For this review, take the finished solid that the model builds, in its own axes (mm). Coordinates: 2 decimals unless noted, no trailing zeros.
```python
from build123d import *

# Parameters (mm, degrees)
MODEL_R             = 2.75
BOSS_EXTRUDE1_DEPTH = 250


with BuildPart() as part:
    # Model → Boss-Extrude1 (new body)
    with BuildSketch(Plane.XY):
        with BuildLine():
            Line((1.499999935, 19.99999323), (6.799999935, 19.99999323))
            Line((6.799999935, 19.99999323), (6.799999935, 18.69999323))
            Line((6.799999935, 18.69999323), (3.999999935, 18.69999323))
            Line((3.999999935, 18.69999323), (3.999999935, 17.19999323))
            Line((3.999999935, 17.19999323), (6.745762647, 14.5))
            Line((6.745762647, 14.5), (9.565216879, 14.5))
            Line((9.565216879, 14.5), (10, 14.25))
            Line((10, 14.25), (10.434782606, 14.5))
            Line((10.434782606, 14.5), (13.254244108, 14.5))
            Line((13.254244108, 14.5), (15.999999935, 17.19999323))
            Line((15.999999935, 17.19999323), (15.999999935, 18.69999323))
            Line((15.999999935, 18.69999323), (13.199999935, 18.69999323))
            Line((13.199999935, 18.69999323), (13.199999935, 19.99999323))
            Line((13.199999935, 19.99999323), (18.499999935, 19.99999323))
            ThreePointArc((18.499999935, 19.99999323), (19.560660107, 19.560653402), (19.999999935, 18.49999323))
            Line((19.999999935, 18.49999323), (19.999999935, 13.19999323))
            Line((19.999999935, 13.19999323), (18.699999935, 13.19999323))
            Line((18.699999935, 13.19999323), (18.699999935, 15.99999323))
            Line((18.699999935, 15.99999323), (17.199999935, 15.99999323))
            Line((17.199999935, 15.99999323), (14.500000065, 13.254230518))
            Line((14.500000065, 13.254230518), (14.500000065, 10.434776138))
            Line((14.500000065, 10.434776138), (14.250000065, 9.99999323))
            Line((14.250000065, 9.99999323), (14.500000065, 9.565210911))
            Line((14.500000065, 9.565210911), (14.500000065, 6.745755942))
            Line((14.500000065, 6.745755942), (17.199999935, 3.99999323))
            Line((17.199999935, 3.99999323), (18.699999935, 3.99999323))
            Line((18.699999935, 3.99999323), (18.699999935, 6.79999323))
            Line((18.699999935, 6.79999323), (19.999999935, 6.79999323))
            Line((19.999999935, 6.79999323), (19.999999935, 1.49999323))
            ThreePointArc((19.999999935, 1.49999323), (19.560660107, 0.439333058), (18.499999935, -6.77e-06))
            Line((18.499999935, -6.77e-06), (13.199999935, -6.77e-06))
            Line((13.199999935, -6.77e-06), (13.199999935, 1.29999323))
            Line((13.199999935, 1.29999323), (15.999999935, 1.29999323))
            Line((15.999999935, 1.29999323), (15.999999935, 2.798703306))
            Line((15.999999935, 2.798703306), (13.254126104, 5.49999323))
            Line((13.254126104, 5.49999323), (10.434782606, 5.49999323))
            Line((10.434782606, 5.49999323), (10, 5.74999323))
            Line((10, 5.74999323), (9.565216879, 5.49999323))
            Line((9.565216879, 5.49999323), (6.745762647, 5.49999323))
            Line((6.745762647, 5.49999323), (3.999999935, 2.79999323))
            Line((3.999999935, 2.79999323), (3.999999935, 1.29999323))
            Line((3.999999935, 1.29999323), (6.799999935, 1.29999323))
            Line((6.799999935, 1.29999323), (6.799999935, -6.77e-06))
            Line((6.799999935, -6.77e-06), (1.499999935, -6.77e-06))
            ThreePointArc((1.499999935, -6.77e-06), (0.439339764, 0.439333058), (-6.5e-08, 1.49999323))
            Line((-6.5e-08, 1.49999323), (-6.5e-08, 6.79999323))
            Line((-6.5e-08, 6.79999323), (1.299999935, 6.79999323))
            Line((1.299999935, 6.79999323), (1.299999935, 3.99999323))
            Line((1.299999935, 3.99999323), (2.799999935, 3.99999323))
            Line((2.799999935, 3.99999323), (5.499999935, 6.745755942))
            Line((5.499999935, 6.745755942), (5.499999935, 9.565210911))
            Line((5.499999935, 9.565210911), (5.749999935, 9.99999323))
            Line((5.749999935, 9.99999323), (5.499999935, 10.434776138))
            Line((5.499999935, 10.434776138), (5.499999935, 13.254230518))
            Line((5.499999935, 13.254230518), (2.799999935, 15.99999323))
            Line((2.799999935, 15.99999323), (1.299999935, 15.99999323))
            Line((1.299999935, 15.99999323), (1.299999935, 13.19999323))
            Line((1.299999935, 13.19999323), (-6.5e-08, 13.19999323))
            Line((-6.5e-08, 13.19999323), (-6.5e-08, 18.49999323))
            ThreePointArc((-6.5e-08, 18.49999323), (0.439339764, 19.560653402), (1.499999935, 19.99999323))
        make_face()
        with Locations((10, 10)):
            Circle(MODEL_R, mode=Mode.SUBTRACT)
    extrude(amount=BOSS_EXTRUDE1_DEPTH)


solid = part.part
```
Q1. Clearance check with flat-ended pins moving along their axes: pin 1 Ø1.5 at (x, z) = (11.5, 187) entering from -Y; pin 2 Ø0.8 at (y, z) = (12, 186) entering from -X; pin 3 Ø2.5 at (y, z) = (8.5, 62.5) entering from +X. State where each tip first meets the part, or that it passes through.
Ans:
pin 1: stops at y = 5.5
pin 2: stops at x = 5.5
pin 3: stops at x = 14.5
Q2. Draft analysis for pull direction X (two halves, no side actions). For faces 1 (the flat face through (0, 16, 123)), 2 (the flat face through (7.9, 7.9, 250)), 3 (the cylindrical face through (11.48, 12.32, 123.25)), 4 (the flat face through (20, 4, 123)), state which applies: +X half, -X half, draft (parallel to the pull), parting line (faces both ways), or undercut.
Ans:
face 1: -X half
face 2: draft
face 3: undercut
face 4: +X half
Q3. For probe 1 along Y at (x, z) = (6.75, 65); probe 2 along X at (y, z) = (5.25, 120.5); probe 3 along Y at (x, z) = (5, 57), list the stretches that pass through material, from the lowest coordinate up.
Ans:
probe 1: y = 0 to 1.3, 5.5 to 14.5, 18.7 to 20
probe 2: x = 0 to 1.3, 4.03 to 6.49, 13.51 to 15.97, 18.7 to 20
probe 3: y = 0 to 1.3, 3.78 to 6.24, 13.76 to 16.22, 18.7 to 20
